CAD build for the part. Positions are in the model's coordinates, mm. Face numbers are marked on the shaded views. A direction names the side the tool comes from. Round coordinates to 2 decimals unless told otherwise and drop trailing zeros. Order: outer loops, then holes, each group sorted by start corner. A loop starts at its lowest first (then second) coordinate and runs counter-clockwise, first axis right, second up. Notation, with made-up numbers: M -18.75,14.5 L 9.25,14.5 A14 ccw 9.25,32.5 Z; hole C 40,12 d1. An arc over 180 degrees is marked long. Answer as a JSON object with one key per item and string values.
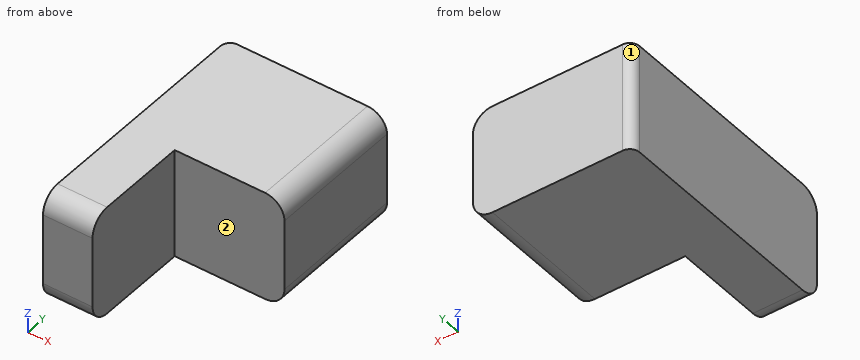
```python
from build123d import *

# Parameters (mm, degrees)
F0_W     = 16.4
F0_H     = 25.4
F1_DEPTH = 11.3
F2_W     = 11.3
F2_H     = 11.3
F3_DEPTH = 25
F4_R     = 2
F5_R     = 1


with BuildPart() as f1:
    # F0 (on Top) → F1 (new body)
    with BuildSketch(Plane.XY):
        with Locations((8.2, 12.7)):
            Rectangle(F0_W, F0_H)
    extrude(amount=F1_DEPTH)

    # F2 (on face) → F3 (cut)
    with BuildSketch(Plane.XY.offset(11.3)):
        with Locations((10.75, 5.65)):
            Rectangle(F2_W, F2_H)
    extrude(amount=-F3_DEPTH, mode=Mode.SUBTRACT)

    # F4
    f4_edges = [f1.edges().sort_by_distance(p)[0] for p in [
        (16.4, 18.35, 0),
        (2.55, 0, 0),
        (2.55, 0, 11.3),
        (16.4, 18.35, 11.3),
    ]]
    fillet(f4_edges, radius=F4_R)

    # F5
    f5_edges = [f1.edges().sort_by_distance(p)[0] for p in [
        (0, 25.4, 5.65),
    ]]
    fillet(f5_edges, radius=F5_R)


solid = f1.part
```
Item 1: Drop a flat-ended pin along its axis: pin 1 Ø3.5 at (x, z) = (10, 4) entering from -Y. Give the stop position or say it passes through.
Worked answers:
{"pin 1": "stops at y = 11.3"}
Item 2: 3-axis set-ups, long thin cutter, end or side, ignore diameter. For the marked faces 1 and 2: which of +Z, -Z, +X, -X, +Y, -Y reach the whole face in a straight line?
Worked answers:
{"face 1": "+Z, -Z, -X, +Y", "face 2": "+Z, -Z, +X, -Y"}
Item 3: Saw through at C-C on x = 10.75. List the corners of the cut face in (y, z), and give its area (3 significant figures).
Worked answers:
{"outline": "M 11.3,0 L 25.4,0 L 25.4,11.3 L 11.3,11.3 Z", "area": "159 mm2"}
Item 4: Saw through at D-D on z = 1.5. List the corners of the cut face in (x, y).
Worked answers:
{"outline": "M 0,0.06 L 5.1,0.06 L 5.1,11.3 L 16.34,11.3 L 16.34,25.4 L 1,25.4 A1 ccw 0,24.4 Z"}
Item 5: Saw through at A-A on z = 6.75. List the corners of the cut face in (x, y), and give its area (3 significant figures).
Worked answers:
{"outline": "M 0,0 L 5.1,0 L 5.1,11.3 L 16.4,11.3 L 16.4,25.4 L 1,25.4 A1 ccw 0,24.4 Z", "area": "289 mm2"}
Item 6: Wall check: line 1 along Y through (x, z) = (7.75, 9.5); line 2 along X through (y, z) = (9.5, 6.5); line 3 along X through (y, z) = (23.25, 1.75). Give the ranges that are in metal, low to high. Write a range as [from, to].
Worked answers:
{"line 1": "y = [11.3, 25.4]", "line 2": "x = [0, 5.1]", "line 3": "x = [0, 16.38]"}
Item 7: Saw through at B-B on y = 7.5. List the corners of the cut face in (x, z), and give its area (3 significant figures).
Worked answers:
{"outline": "M 0,0 L 5.1,0 L 5.1,11.3 L 0,11.3 Z", "area": "57.6 mm2"}
